Part model, mm, in its own coordinate system. Face numbers are marked on the shaded views. A direction names the side the tool comes from. Coordinates: 2 decimals unless noted, no trailing zeros. Order: outer loops, then holes, each group sorted by start corner. A loop starts at its lowest first (then second) coordinate and runs counter-clockwise, first axis right, second up.
1) Pin check, flat tips, straight feed: pin 1 Ø16.5 at (x, y) = (4.5, 1) entering from +Z; pin 2 Ø1.5 at (x, z) = (-10.5, 20.5) entering from +Y; pin 3 Ø8 at (x, y) = (-3, 0) entering from +Z; pin 4 Ø1.5 at (x, z) = (-1, 14) entering from -Y. Stop position of each tip, or through.
2) Mould opens along Z. For the marked faces 1, 2 and 3 say: +Z half, -Z half, draft (parallel to the pull), parting line (faces both ways), or undercut.
3) Cut at B-B (x = -10). List the corners of the cut face in (y, z), and give its area (3 significant figures).
4) Wall check: L1, parallel to Z at x = -3.25, y = -6.75; L2, parallel to Y at x = 0, z = 45.5; L3, parallel to Z at x = 3.5, y = -0.5. Give the ranges that are in metal, low to high.
5) Cut at C-C (y = -2). List the corners of the cut face in (x, z).
6) Cut at D-D (z = -13.5). List the corners of the cut face in (x, y), and give its area (3 significant figures).
7) Tool access for the marked faces 4, 5 and 6: list every direction of +Z, -Z, +X, -X, +Y, -Y with a clear straight run to the whole face (end or side of a thin tool).
8) Cut at A-A (z = 60.5). List the corners of the cut face in (x, y).
```python
from build123d import *

# Parameters (mm, degrees)
ESQUISSE1_R             = 15
BOSS_EXTRU_1_DEPTH      = 70
ESQUISSE2_R             = 12
ENL_V_MAT_EXTRU_1_DEPTH = 65
ESQUISSE3_W             = 5
ESQUISSE3_H             = 15
BOSS_EXTRU_2_DEPTH      = 5
ESQUISSE12_W            = 5
ESQUISSE12_H            = 15
BOSS_EXTRU_6_DEPTH      = 10
ESQUISSE13_W            = 5
ESQUISSE13_H            = 15
BOSS_EXTRU_7_DEPTH      = 15
ESQUISSE14_W            = 4.52084763
ESQUISSE14_H            = 15
BOSS_EXTRU_8_DEPTH      = 15


with BuildPart() as part:
    # Esquisse1 → Boss.-Extru.1 (new body)
    with BuildSketch(Plane.XY):
        Circle(ESQUISSE1_R)
    extrude(amount=BOSS_EXTRU_1_DEPTH)

    # Esquisse2 → Enlèv. mat.-Extru.1 (cut)
    with BuildSketch(Plane.XY.offset(70)):
        Circle(ESQUISSE2_R)
    extrude(amount=-ENL_V_MAT_EXTRU_1_DEPTH, mode=Mode.SUBTRACT)

    # Esquisse3 → Boss.-Extru.2 (add)
    with BuildSketch(Plane(origin=(0, 0, 0), x_dir=(-1, 0, 0), z_dir=(0, 0, -1))):
        with Locations((-2.5, 0)):
            Rectangle(ESQUISSE3_W, ESQUISSE3_H)
    extrude(amount=BOSS_EXTRU_2_DEPTH)

    # Esquisse12 → Boss.-Extru.6 (add)
    with BuildSketch(Plane(origin=(5, 0, 0), x_dir=(0, 0, -1), z_dir=(1, 0, 0))):
        with Locations((2.5, 0)):
            Rectangle(ESQUISSE12_W, ESQUISSE12_H)
    extrude(amount=BOSS_EXTRU_6_DEPTH)

    # Esquisse13 → Boss.-Extru.7 (add)
    with BuildSketch(Plane(origin=(0, 0, -5), x_dir=(-1, 0, 0), z_dir=(0, 0, -1))):
        with Locations((-12.5, 0)):
            Rectangle(ESQUISSE13_W, ESQUISSE13_H)
    extrude(amount=BOSS_EXTRU_7_DEPTH)

    # Esquisse14 → Boss.-Extru.8 (add)
    with BuildSketch(Plane.ZY.offset(-10)):
        with Locations((-17.739576185, 0)):
            Rectangle(ESQUISSE14_W, ESQUISSE14_H)
    extrude(amount=BOSS_EXTRU_8_DEPTH)


solid = part.part
```
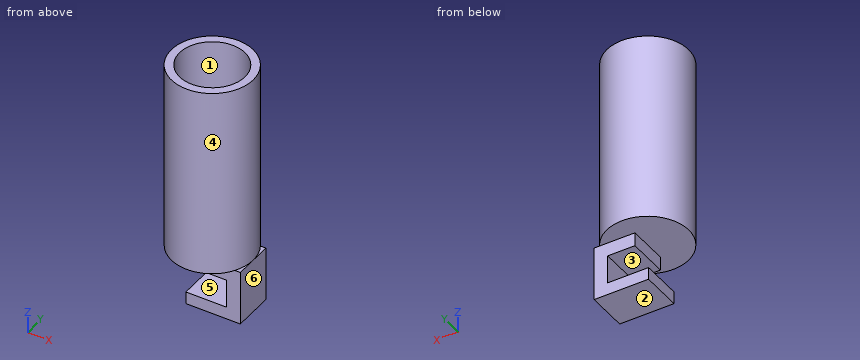
Geometry check:
1. pin 1: stops at z = 70
1. pin 2: stops at y = 11.4
1. pin 3: stops at z = 5
1. pin 4: stops at y = -15
2. face 1: draft
2. face 2: -Z half
2. face 3: undercut
3. outline: (-11.18, 0) - (11.18, 0) - (11.18, 70) - (6.63, 70) - (6.63, 5) - (-6.63, 5) - (-6.63, 70) - (-11.18, 70) - close
3. area: 703 mm2
4. L1: z = -20 to -15.48, 0 to 5
4. L2: y = -15 to -12, 12 to 15
4. L3: z = -20 to -15.48, -5 to 5
5. outline: (-14.87, 0) - (0, 0) - (0, -5) - (10, -5) - (10, -15.48) - (-5, -15.48) - (-5, -20) - (15, -20) - (15, 0) - (14.87, 0) - (14.87, 70) - (11.83, 70) - (11.83, 5) - (-11.83, 5) - (-11.83, 70) - (-14.87, 70) - close
6. outline: (10, -7.5) - (15, -7.5) - (15, 7.5) - (10, 7.5) - close
6. area: 75.0 mm2
7. face 4: +Z
7. face 5: -X, +Y, -Y
7. face 6: +Z, -Z, +X, +Y, -Y
8. outline: circle Ø30 at (0, 0); hole circle Ø24 at (0, 0)
